```python
from build123d import *

# Parameters (mm, degrees)
F0_R     = 11.684
F1_DEPTH = 78.74
F2_R     = 10.16
F3_DEPTH = 76.2
F4_DEPTH = 2.54
F5_DEPTH = 7.62
F7_DEPTH = 7.62
F6_R     = 10.795
F6_R_2   = 10.16
F9_DEPTH = 12.7


with BuildPart() as f1:
    # F0 (on Top) → F1 (new body)
    with BuildSketch(Plane.XY):
        Circle(F0_R)
    extrude(amount=F1_DEPTH)

    # F2 (on face) → F3 (cut)
    with BuildSketch(Plane.XY.offset(78.74)):
        Circle(F2_R)
    extrude(amount=-F3_DEPTH, mode=Mode.SUBTRACT)

    # F4 (add): a face of the model
    f4_faces = [f1.faces().sort_by_distance(p)[0] for p in [
        (0, 0, 0),
    ]]
    extrude(f4_faces, amount=F4_DEPTH)

    # F5 (add): a face of the model
    f5_faces = [f1.faces().sort_by_distance(p)[0] for p in [
        (0, 0, -2.54),
    ]]
    extrude(f5_faces, amount=F5_DEPTH)

    # F7 (cut): a face of the model
    f7_faces = [f1.faces().sort_by_distance(p)[0] for p in [
        (0, 0, -10.16),
    ]]
    extrude(f7_faces, amount=-F7_DEPTH, mode=Mode.SUBTRACT)

    # F6 (on face) → F9 (join)
    with BuildSketch(Plane.XY.offset(78.74)):
        Circle(F6_R)
        Circle(F6_R_2, mode=Mode.SUBTRACT)
    extrude(amount=F9_DEPTH)


solid = f1.part
```
Can you work these out from the model? Positions are in its coordinate system, mm. A direction names the side the tool comes from. Give positions to 0.01 mm unless a question says otherwise; leave off trailing zeros. Loops run counter-clockwise (first coordinate to the right, second up) from the corner with the lowest first, then second, coordinate; pieces in that order, holes last. Notation, with made-up numbers: M -18.75,65 L -10.75,65 A13 ccw -10.75,72 Z; hole C 42.25,69 d7. An arc over 180 degrees is marked long. Use one line per item in the form item = value. Start each with the question number.
(1) I'm going to push flat-ended pins straight in: P1, Ø1, axis at x = 6, z = 77, coming from the -Y side; P2, Ø5, axis at y = -6, z = 14, coming from the +X side; P3, Ø5, axis at x = -2, y = -1.5, coming from the +Z side. Where does each tip first touch, or does it pass through?
(2) On a 3-axis mill with a long thin cutter (end or side, diameter ignored), from which of +Z, -Z, +X, -X, +Y, -Y can I reach the whole of each face in a straight line? I mean faces 1 (the cylindrical face through (-7.956, 7.296, 85.001)), 2 (the flat face through (3.95, -9.55, 91.44)). Say none if no direction works.
(3) Please list where these lines run through material, in increasing order: line 1 (Z direction, x = 8.75, y = -3.5); line 2 (Y direction, x = 0, z = 72); line 3 (X direction, y = 2, z = 21).
(4) Thinking about a two-plate mould opening in X: for faces 3 (the cylindrical face through (-2.533, -11.406, 38.669)), 4 (the flat face through (8, -8, 78.74)), 5 (the cylindrical face through (-1.323, 10.074, 46.368)), which applies, released by +X, released by -X, zero draft, split by the parting line, or undercut?
(5) I want a section at A-A, the plane x = 0. Write out the boundary of the cut face in (y, z) (3 decimals).
(6) I want a section at C-C, the plane z = 53. Write out the boundary of the cut face in (x, y).
Worked out:
q1.P1 = -10.31
q1.P2 = 11.15
q1.P3 = 2.54
q2.face_1 = +Z
q2.face_2 = +Z, +X, -X, +Y, -Y
q3.line_1 = -2.54 to 2.54
q3.line_2 = -11.68 to -10.16, 10.16 to 11.68
q3.line_3 = -11.51 to -9.96, 9.96 to 11.51
q4.face_3 = split by the parting line
q4.face_4 = zero draft
q4.face_5 = undercut
q5.outline = M -11.684,-2.54 L 11.684,-2.54 L 11.684,78.74 L 10.795,78.74 L 10.795,91.44 L 10.16,91.44 L 10.16,2.54 L -10.16,2.54 L -10.16,91.44 L -10.795,91.44 L -10.795,78.74 L -11.684,78.74 Z
q6.outline = C 0,0 d23.37; hole C 0,0 d20.32
